Geometry: final body of the model. Coordinates: model frame, mm. A direction names the side the tool comes from. Coordinates: 2 decimals unless noted, no trailing zeros. Write each loop counter-clockwise with the first axis right and the second up, starting at its lowest first coordinate (ties: lowest second). Pieces come first, ordered by that corner, then holes. Notation, with made-up numbers: (61, 23.25) -> (95, 23.25) arc R7 ccw to (95, 35.25) -> close; hole circle Ø9 at (17, 15.5). An arc over 180 degrees is marked (long way). One line per item, written item: value.
```python
from build123d import *

# Parameters (mm, degrees)
SKETCH1_R                        = 12.5
SKETCH1_R_2                      = 5.65
BOSS_EXTRUDE1_DEPTH              = 60
F_6_0MM_DOWEL_HOLE1_D            = 5.4
F_6_0MM_DOWEL_HOLE1_DEPTH        = 10
TAP_DRILL_FOR_M3_HELICOIL1_D     = 3.15
TAP_DRILL_FOR_M3_HELICOIL1_DEPTH = 10
BOSS_EXTRUDE2_START              = 7
SKETCH17_R                       = 12.5
BOSS_EXTRUDE2_DEPTH              = 7
SKETCH18_R                       = 3.5
BOSS_EXTRUDE3_DEPTH              = 10
SKETCH20_W                       = 1.65
SKETCH20_H                       = 10
F_3_0MM_DOWEL_HOLE2_D            = 3.3
SKETCH24_R                       = 1.65
SKETCH27_R                       = 1.65
F_6_0MM_DOWEL_HOLE2_REACH        = 71.293
F_6_0MM_DOWEL_HOLE2_BORE_R       = 1.65
F_6_0MM_DOWEL_HOLE3_REACH        = 71.293
F_6_0MM_DOWEL_HOLE3_BORE_R       = 1.65
F_6_0MM_DOWEL_HOLE4_D            = 3
F_6_0MM_DOWEL_HOLE4_DEPTH        = 10


with BuildPart() as part:
    # Sketch1 → Boss-Extrude1 (new body)
    with BuildSketch(Plane(origin=(0, 0, 0), x_dir=(1, 0, 0), z_dir=(0, 1, 0))):
        with Locations(Location((0, 0, 0), (0, 0, 270))):
            Circle(SKETCH1_R)
        with Locations(Location((3, 0, 0), (0, 0, 270))):
            Circle(SKETCH1_R_2, mode=Mode.SUBTRACT)
    extrude(amount=BOSS_EXTRUDE1_DEPTH)

    # Ø6.0mm Dowel Hole1
    with Locations(Plane(origin=(0, 60, 0), x_dir=(1, 0, 0), z_dir=(0, 1, 0))):
        with Locations((-5.462566323, 5.462566323), (-5.462566323, -5.462566323)):
            Hole(F_6_0MM_DOWEL_HOLE1_D / 2, depth=F_6_0MM_DOWEL_HOLE1_DEPTH)

    # Tap Drill for M3 Helicoil1
    with Locations(Plane(origin=(0, 60, 0), x_dir=(1, 0, 0), z_dir=(0, 1, 0))):
        with Locations((4.75, 8.227241336), (4.75, -8.227241336), (-9.5, 0)):
            Hole(TAP_DRILL_FOR_M3_HELICOIL1_D / 2, depth=TAP_DRILL_FOR_M3_HELICOIL1_DEPTH)

    # Sketch17 → Boss-Extrude2 (add)
    with BuildSketch(Plane.XZ.offset(BOSS_EXTRUDE2_START)):
        with Locations(Location((0, 0, 0), (0, 0, 270))):
            Circle(SKETCH17_R)
    extrude(amount=-BOSS_EXTRUDE2_DEPTH)

    # Sketch18 → Boss-Extrude3 (add)
    with BuildSketch(Plane.XZ.offset(7)):
        with Locations(Location((0, 0, 0), (0, 0, 270))):
            Circle(SKETCH18_R)
    extrude(amount=BOSS_EXTRUDE3_DEPTH)

    # Sketch20 → Ø3.0mm Dowel Hole1 (revolve, cut)
    with BuildSketch(Plane(origin=(0, -7, 0), x_dir=(0, 0, 1), z_dir=(1, 0, 0))):
        with Locations((0.825, 5)):
            Rectangle(SKETCH20_W, SKETCH20_H)
    revolve(axis=Axis((0, -0.65, 0), (0, -1, 0)), mode=Mode.SUBTRACT)

    # Ø3.0mm Dowel Hole2 (through all)
    with Locations(Plane(origin=(0, 0, 0), x_dir=(1, 0, 0), z_dir=(0, 1, 0))):
        with Locations((0, 0)):
            Hole(F_3_0MM_DOWEL_HOLE2_D / 2)

    # Cut-Sweep5: sweep along a curve in space
    with BuildLine() as cut_sweep5_path:
        Line((0, 24.869183639, 0), (-8.875394659, 37.420887137, -8.875394659))
    # Sketch24 → Cut-Sweep5 (sweep, cut)
    with BuildSketch(Plane(origin=(-8.838834765, 0, -8.838834765), x_dir=(-0.7071067811865462, 0, 0.7071067811865488), z_dir=(-0.7071067811865488, 0, -0.7071067811865462))):
        with Locations((0, 36.882111372)):
            Circle(SKETCH24_R)
    sweep(path=cut_sweep5_path.line, mode=Mode.SUBTRACT)

    # Cut-Sweep6: sweep along a curve in space
    with BuildLine() as cut_sweep6_path:
        Line((-3.623287534, 30, 3.623287534), (-12.526142338, 42.590538007, 12.526142338))
        Line((-3.623287534, 30, 3.623287534), (0, 24.875897629, 0))
    # Sketch27 → Cut-Sweep6 (sweep, cut)
    with BuildSketch(Plane(origin=(-8.838834765, 0, 8.838834765), x_dir=(0.7071067811865488, 0, 0.7071067811865462), z_dir=(-0.7071067811865462, 0, 0.7071067811865488))):
        with Locations((0, 36.98969213)):
            Circle(SKETCH27_R)
    sweep(path=cut_sweep6_path.line, mode=Mode.SUBTRACT)

    # Ø6.0mm Dowel Hole2 bore → Ø6.0mm Dowel Hole2 (cut, up to next)
    with BuildSketch(Plane(origin=(0, 50, 0), x_dir=(1, 0, 0), z_dir=(0, 1, 0)), mode=Mode.PRIVATE) as f_6_0mm_dowel_hole2_sk1:
        with Locations((-5.462566323, 5.462566323)):
            Circle(F_6_0MM_DOWEL_HOLE2_BORE_R)
    f_6_0mm_dowel_hole2_tool1 = extrude(f_6_0mm_dowel_hole2_sk1.sketch, amount=-F_6_0MM_DOWEL_HOLE2_REACH, mode=Mode.PRIVATE) & part.part
    add(f_6_0mm_dowel_hole2_tool1.solids().sort_by_distance((-5.462566, 50, -5.462566))[0], mode=Mode.SUBTRACT)

    # Ø6.0mm Dowel Hole3 bore → Ø6.0mm Dowel Hole3 (cut, up to next)
    with BuildSketch(Plane(origin=(0, 50, 0), x_dir=(1, 0, 0), z_dir=(0, 1, 0)), mode=Mode.PRIVATE) as f_6_0mm_dowel_hole3_sk1:
        with Locations((-5.462566323, -5.462566323)):
            Circle(F_6_0MM_DOWEL_HOLE3_BORE_R)
    f_6_0mm_dowel_hole3_tool1 = extrude(f_6_0mm_dowel_hole3_sk1.sketch, amount=-F_6_0MM_DOWEL_HOLE3_REACH, mode=Mode.PRIVATE) & part.part
    add(f_6_0mm_dowel_hole3_tool1.solids().sort_by_distance((-5.462566, 50, 5.462566))[0], mode=Mode.SUBTRACT)

    # Ø6.0mm Dowel Hole4
    with Locations(Plane(origin=(0, -7, 0), x_dir=(-1, 0, 0), z_dir=(0, -1, 0))):
        with Locations((-4.5, -7.794228634), (9, 0), (-4.5, 7.794228634)):
            Hole(F_6_0MM_DOWEL_HOLE4_D / 2, depth=F_6_0MM_DOWEL_HOLE4_DEPTH)


solid = part.part
```
(1) Section B-B (x = 4.5). Return the cut outline in (y, z).
Responses:
outline: (-7, -11.66) -> (60, -11.66) -> (60, -9.78) -> (50, -9.78) -> (50, -6.67) -> (60, -6.67) -> (60, -5.45) -> (0, -5.45) -> (0, 5.45) -> (60, 5.45) -> (60, 6.67) -> (50, 6.67) -> (50, 9.78) -> (60, 9.78) -> (60, 11.66) -> (-7, 11.66) -> (-7, 9.29) -> (3, 9.29) -> (3, 6.29) -> (-7, 6.29) -> (-7, -6.29) -> (3, -6.29) -> (3, -9.29) -> (-7, -9.29) -> close
(2) Pull-direction query (Z, two-part tool) for faces 4 (the flat face through (-3, 60, 3)), 5 (the flat face through (5, 50, -8)), 6 (the cylindrical face through (-3.417, -11.93, 0.759)); classes: released by +Z, released by -Z, zero draft, split by the parting line, or undercut.
Responses:
face 4: zero draft
face 5: undercut
face 6: split by the parting line
(3) Line query: line 1 (X direction, y = 21.5, z = 0); line 2 (Z direction, x = 4.5, y = -3.5); line 3 (Z direction, x = 0, y = -5.25). Output: solid intervals per line, ascending. Write a range as [from, to].
Responses:
line 1: x = [-12.5, -2.65], [8.65, 12.5]
line 2: z = [-11.66, -9.29], [-6.29, 6.29], [9.29, 11.66]
line 3: z = [-12.5, -1.65], [1.65, 12.5]
(4) Section A-A (y = 7.5). Return the cut outline in (x, z).
Responses:
outline: circle Ø25 at (0, 0); hole circle Ø11.3 at (3, 0)
(5) First-contact query: pin 1 (2.5 mm diameter, centred on x = 4.75, z = 8.23, fed in from +Y); pin 2 (4.5 mm diameter, centred on x = 0, z = 0, fed in from +Y); pin 3 (1.5 mm diameter, centred on x = 4, z = -7, fed in from -Y). Flat tips, straight axial feed; report the tip coordinate or a pass-through.
Responses:
pin 1: stops at y = 50
pin 2: stops at y = 0
pin 3: stops at y = -7
(6) Reachability of faces 1 (the cylindrical face through (-4.58, 41.23, 4.07)), 2 (the flat face through (-1, -17, -2)), 3 (the cylindrical face through (-10.5, -1.93, -0.07)) from +Z, -Z, +X, -X, +Y, -Y: full face, straight path, thin tool, end or side. Return the list, or none.
Responses:
face 1: +Y
face 2: +Z, -Z, +X, -X, -Y
face 3: -Y
(7) Section C-C (y = 41). Return the cut outline in (x, z).
Responses:
outline: circle Ø25 at (0, 0); hole circle Ø3.3 at (-5.46, -5.46); hole circle Ø3.3 at (-5.46, 5.46); hole circle Ø11.3 at (3, 0)
